from build123d import *

# Parameters (mm, degrees)
F1_DEPTH = 5
F2_R     = 5
F3_R     = 0.99999


# Not quite as in the source:
# - a fillet or chamfer is up to 0.001 mm smaller than in the source, because OpenCascade refuses the exact size


with BuildPart() as f1:
    # F0 (on Top) → F1 (new body)
    with BuildSketch(Plane.XY):
        with BuildLine():
            ThreePointArc((5.4121153846, -14.9505520655), (-15.9, 0), (5.4121153846, 14.9505520655))
            Line((5.4121153846, 14.9505520655), (13.1430758683, 12.1519363363))
            ThreePointArc((13.1430758683, 12.1519363363), (9.898446583, 14.91411262), (6.0928846154, 16.8311246524))
            ThreePointArc((6.0928846154, 16.8311246524), (-17.9, 0), (6.0928846154, -16.8311246524))
            ThreePointArc((6.0928846154, -16.8311246524), (9.898446583, -14.91411262), (13.1430758683, -12.1519363363))
            Line((13.1430758683, -12.1519363363), (5.4121153846, -14.9505520655))
        make_face()
        with BuildLine():
            ThreePointArc((6.0928846154, 16.8311246524), (9.898446583, 14.91411262), (13.1430758683, 12.1519363363))
            Line((13.1430758683, 12.1519363363), (36.3130060827, 3.76439752))
            ThreePointArc((36.3130060827, 3.76439752), (38.3715715504, 4.5821067953), (40.5742788462, 4.3488241071))
            Line((40.5742788462, 4.3488241071), (6.0928846154, 16.8311246524))
        make_face()
        with BuildLine():
            Line((36.3130060827, -3.76439752), (13.1430758683, -12.1519363363))
            ThreePointArc((13.1430758683, -12.1519363363), (9.898446583, -14.91411262), (6.0928846154, -16.8311246524))
            Line((6.0928846154, -16.8311246524), (40.5742788462, -4.3488241071))
            ThreePointArc((40.5742788462, -4.3488241071), (38.3715715504, -4.5821067953), (36.3130060827, -3.76439752))
        make_face()
        with BuildLine():
            ThreePointArc((40.5742788462, 4.3488241071), (38.3715715504, 4.5821067953), (36.3130060827, 3.76439752))
            Line((36.3130060827, 3.76439752), (39.8935096154, 2.4682515202))
            ThreePointArc((39.8935096154, 2.4682515202), (41.1489634409, 1.507508252), (41.625, 0))
            ThreePointArc((41.625, 0), (41.1489634409, -1.507508252), (39.8935096154, -2.4682515202))
            Line((39.8935096154, -2.4682515202), (36.3130060827, -3.76439752))
            ThreePointArc((36.3130060827, -3.76439752), (38.3715715504, -4.5821067953), (40.5742788462, -4.3488241071))
            ThreePointArc((40.5742788462, -4.3488241071), (42.7862689196, -2.6560859678), (43.625, 0))
            ThreePointArc((43.625, 0), (42.7862689196, 2.6560859678), (40.5742788462, 4.3488241071))
        make_face()
        with BuildLine():
            Line((39.8935096154, 2.4682515202), (36.3130060827, 3.76439752))
            ThreePointArc((36.3130060827, 3.76439752), (34.375, 0), (36.3130060827, -3.76439752))
            Line((36.3130060827, -3.76439752), (39.8935096154, -2.4682515202))
            ThreePointArc((39.8935096154, -2.4682515202), (36.375, 0), (39.8935096154, 2.4682515202))
        make_face()
        with BuildLine():
            ThreePointArc((5.4121153846, 14.9505520655), (13.0165785561, 9.1311928406), (15.9, 0))
            ThreePointArc((15.9, 0), (13.0165785561, -9.1311928406), (5.4121153846, -14.9505520655))
            Line((5.4121153846, -14.9505520655), (13.1430758683, -12.1519363363))
            ThreePointArc((13.1430758683, -12.1519363363), (16.6683991139, -6.5249115687), (17.9, 0))
            ThreePointArc((17.9, 0), (16.6683991139, 6.5249115687), (13.1430758683, 12.1519363363))
            Line((13.1430758683, 12.1519363363), (5.4121153846, 14.9505520655))
        make_face()
    extrude(amount=F1_DEPTH)

    # F2
    f2_edges = [f1.edges().sort_by_distance(p)[0] for p in [
        (36.313006, 3.764398, 2.5),
        (36.313006, -3.764398, 2.5),
        (13.143076, 12.151936, 2.5),
        (13.143076, -12.151936, 2.5),
    ]]
    fillet(f2_edges, radius=F2_R)

    # F3 (radius 1 in the source; OpenCascade refuses exactly that, so slightly less here)
    f3_edges = [f1.edges().sort_by_distance(p)[0] for p in [
        (23.333582, 10.589974, 5),
        (19.479429, 7.262513, 5),
    ]]
    fillet(f3_edges, radius=F3_R)


solid = f1.part
Input: part model. Units: mm. Frame: model coordinates. A direction names the side the tool comes from. Coordinates: 2 decimals unless noted, no trailing zeros. One line per question, with ' | ' between items.
Item 1: Draft query along Y for faces 1 (the flat face through (27.689, 6.886, 1.972)), 2 (the flat face through (23.575, 10.503, 1.972)), 3 (the flat face through (23.09, -10.68, 1.97)), 4 (the cylindrical face through (33.675, -3.57, 2.028)). Return one class per face: released by +Y, released by -Y, zero draft, split by the parting line, or undercut.
Geometry results:
face 1: undercut | face 2: released by +Y | face 3: released by -Y | face 4: undercut
Item 2: Reachability of faces 5 (the cylindrical face through (27.88, -7.12, 4.7)), 6 (the flat face through (27.783, -6.852, 1.972)), 7 (the flat face through (17, 1, 0)) from +Z, -Z, +X, -X, +Y, -Y: full face, straight path, thin tool, end or side. Return the list, or none.
Geometry results:
face 5: +Z | face 6: +Z, -Z | face 7: -Z, +X, -X, +Y, -Y
Item 3: Pin query (flat end, axial travel): pin 1 (2 mm diameter, centred on y = 3.5, z = 4, fed in from +X). Return the tip coordinate at first contact, or that it passes through.
Geometry results:
pin 1: stops at x = 42.89
Item 4: Ray query, line 1 along Y through (x, z) = (0, 1.3); line 2 along X through (y, z) = (-1, 2.8); line 3 along X through (y, z) = (4, 3.8). Return the intervals inside material, ascending.
Geometry results:
line 1: y = -17.9 to -15.9, 15.9 to 17.9 | line 2: x = -17.87 to -15.87, 15.87 to 17.87, 34.42 to 36.57, 41.43 to 43.52 | line 3: x = -17.45 to -15.39, 15.39 to 17.68, 33.38 to 41.32
Item 5: Section A-A (z = 0.9). Give the number of separate pieces and of enclosed holes in the cut face, then the cut area to 3 significant figures.
Geometry results:
separate pieces: 1 | enclosed holes: 3 | area: 429 mm^2
